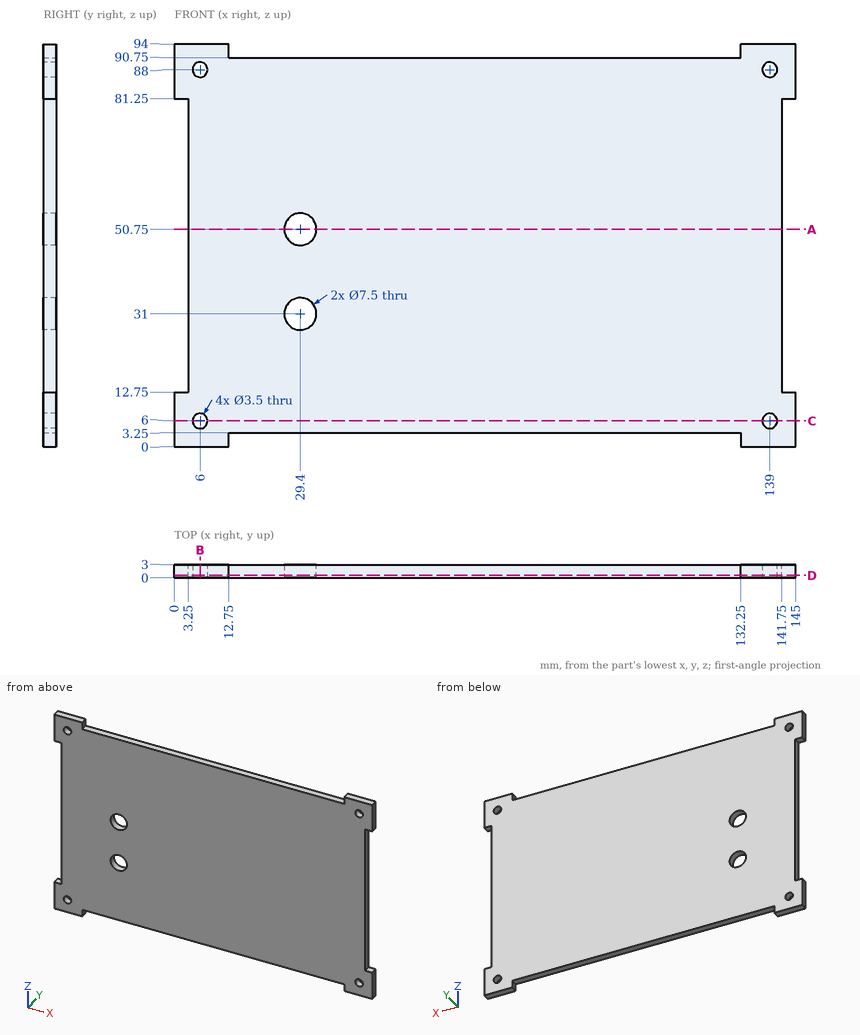
Could you check a few things on this drawing? It's one solid part, dimensions in mm from its lowest x, y, z. Give positions to 0.01 mm unless a question says otherwise; leave off trailing zeros. Order: outer loops, then holes, each group sorted by start corner. A loop starts at its lowest first (then second) coordinate and runs counter-clockwise, first axis right, second up. Notation, with made-up numbers: (-31, -27) - (7, -27) arc R12 ccw to (7, -9) - close; hole circle Ø3 at (-8.5, 67.5). An arc over 180 degrees is marked (long way). One line per item, written item: value. Start each with the question number.
1. Imagine slicing it at C-C on z = 6. List the corners of the cut face in (x, y) for me, plus the area to 3 significant figures.
2. For P1, Ø1, axis at y = 2.5, z = 49.5, coming from the -X side; P2, Ø1.5, axis at y = 1.5, z = 54.5, coming from the +X side, each with a flat end and sliding along its axis, tell me the tip position at first contact or that it passes through.
3. If I drill on probe 1 along Z at (x, y) = (29.4, 1.6); probe 2 along Z at (x, y) = (6, 2.1); probe 3 along X at (y, z) = (1.1, 88), over which ranges is the centre line in solid material (lowest first)?
4. Imagine slicing it at D-D on y = 0.5. List the corners of the cut face in (x, z) for me.
5. Imagine slicing it at B-B on x = 6. List the corners of the cut face in (y, z) for me.
6. Imagine slicing it at A-A on z = 50.75. List the corners of the cut face in (x, y) for me, plus the area to 3 significant figures.
Values:
1. outline: (0, 0) - (4.25, 0) - (4.25, 3) - (0, 3) - close; (7.75, 0) - (137.25, 0) - (137.25, 3) - (7.75, 3) - close; (140.75, 0) - (145, 0) - (145, 3) - (140.75, 3) - close
1. area: 414 mm²
2. P1: x = 3.25
2. P2: x = 141.75
3. probe 1: 3.25 to 27.25, 34.75 to 47, 54.5 to 90.75
3. probe 2: 0 to 4.25, 7.75 to 86.25, 89.75 to 94
3. probe 3: 0 to 4.25, 7.75 to 137.25, 140.75 to 145
4. outline: (0, 0) - (12.75, 0) - (12.75, 3.25) - (132.25, 3.25) - (132.25, 0) - (145, 0) - (145, 12.75) - (141.75, 12.75) - (141.75, 81.25) - (145, 81.25) - (145, 94) - (132.25, 94) - (132.25, 90.75) - (12.75, 90.75) - (12.75, 94) - (0, 94) - (0, 81.25) - (3.25, 81.25) - (3.25, 12.75) - (0, 12.75) - close; hole circle Ø3.5 at (6, 6); hole circle Ø3.5 at (6, 88); hole circle Ø7.5 at (29.4, 31); hole circle Ø7.5 at (29.4, 50.75); hole circle Ø3.5 at (139, 6); hole circle Ø3.5 at (139, 88)
5. outline: (0, 0) - (3, 0) - (3, 4.25) - (0, 4.25) - close; (0, 7.75) - (3, 7.75) - (3, 86.25) - (0, 86.25) - close; (0, 89.75) - (3, 89.75) - (3, 94) - (0, 94) - close
6. outline: (3.25, 0) - (25.65, 0) - (25.65, 3) - (3.25, 3) - close; (33.15, 0) - (141.75, 0) - (141.75, 3) - (33.15, 3) - close
6. area: 393 mm²
